Read the model definition and answer for the solid it produces. Units are mm, in the model's axes. A direction names the side the tool comes from. Round coordinates to 2 decimals unless told otherwise and drop trailing zeros. Order: outer loops, then holes, each group sorted by start corner. A loop starts at its lowest first (then second) coordinate and runs counter-clockwise, first axis right, second up. Notation, with made-up numbers: M 45,5 L 89,5 A13 ccw 89,9 Z; hole C 33.25,41 d8. An arc over 180 degrees is marked long. Answer as CSV lines item,"result".
```python
from build123d import *

# Parameters (mm, degrees)
SKETCH_1_W          = 36
SKETCH_1_H          = 15
EXTRUDE_1_DEPTH     = 4
SKETCH_2_W          = 36
SKETCH_2_H          = 3
EXTRUDE_2_DEPTH     = 10
SKETCH_3_R          = 1.7
CUT_EXTRUDE_1_DEPTH = 8
CHAMFER_1_SIZE      = 2
FILLET_1_R          = 0.5
FILLET_2_R          = 0.5


with BuildPart() as part:
    # Эскиз1 → Бобышка-Вытянуть1 (new body)
    with BuildSketch(Plane(origin=(0, 0, 0), x_dir=(1, 0, 0), z_dir=(0, 1, 0))):
        Rectangle(SKETCH_1_W, SKETCH_1_H)
    extrude(amount=EXTRUDE_1_DEPTH)

    # Эскиз2 → Бобышка-Вытянуть2 (add)
    with BuildSketch(Plane(origin=(0, 4, 0), x_dir=(1, 0, 0), z_dir=(0, 1, 0))):
        with Locations((0, 6)):
            Rectangle(SKETCH_2_W, SKETCH_2_H)
    extrude(amount=EXTRUDE_2_DEPTH)

    # Эскиз3 → Вырез-Вытянуть1 (cut)
    with BuildSketch(Plane.XZ):
        with Locations(Location((15, 0, 0), (0, 0, 270))):
            Circle(SKETCH_3_R)
        with Locations(Location((-15, 0, 0), (0, 0, 270))):
            Circle(SKETCH_3_R)
    extrude(amount=-CUT_EXTRUDE_1_DEPTH, mode=Mode.SUBTRACT)

    # Фаска1
    # the kernel refuses this chamfer: 2 mm, written as the material it takes off along each edge
    with BuildSketch(Plane(origin=(15, 0, 0), x_dir=(0, 0, -1), z_dir=(-1, 0, 0))) as chamfer_1_piece_1:
        Polygon((1.7 + CHAMFER_1_SIZE, 0), (1.7, -CHAMFER_1_SIZE), (1.7, 0), align=None)
    revolve(axis=Axis((15, 0, 0), (0, -1, 0)), mode=Mode.SUBTRACT)
    with BuildSketch(Plane(origin=(-15, 0, 0), x_dir=(0, 0, -1), z_dir=(-1, 0, 0))) as chamfer_1_piece_2:
        Polygon((1.7 + CHAMFER_1_SIZE, 0), (1.7, -CHAMFER_1_SIZE), (1.7, 0), align=None)
    revolve(axis=Axis((-15, 0, 0), (0, -1, 0)), mode=Mode.SUBTRACT)
    with BuildSketch(Plane(origin=(-23.143365976, 0, 7.5), x_dir=(0, 0.9996219169112968, 0.027495876610586494), z_dir=(1, 0, 0))) as chamfer_1_piece_3:
        Polygon((CHAMFER_1_SIZE * 0.999621916911, -CHAMFER_1_SIZE * 0.0274958766106), (-CHAMFER_1_SIZE * 0.0274958766106, -CHAMFER_1_SIZE * 0.999621916911), (0, 0), align=None)
    extrude(amount=46.286731952, mode=Mode.SUBTRACT)
    with BuildSketch(Plane(origin=(-18, 0, -12.643365976), x_dir=(-0.02749587661058563, 0.9996219169112968, 0), z_dir=(0, 0, 1)), Plane(origin=(18, 0, 12.643365976), x_dir=(0.02749587661058563, 0.9996219169112968, 0), z_dir=(0, 0, -1))) as chamfer_1_piece_4:
        Polygon((CHAMFER_1_SIZE * 0.999621916911, -CHAMFER_1_SIZE * 0.0274958766106), (-CHAMFER_1_SIZE * 0.0274958766106, -CHAMFER_1_SIZE * 0.999621916911), (0, 0), align=None)
    extrude(amount=25.286731952, mode=Mode.SUBTRACT)
    with BuildSketch(Plane(origin=(23.143365976, 0, -7.5), x_dir=(0, -0.027495876610586365, 0.9996219169112968), z_dir=(-1, 0, 0))) as chamfer_1_piece_5:
        Polygon((CHAMFER_1_SIZE * 0.999621916911, CHAMFER_1_SIZE * 0.0274958766106), (-CHAMFER_1_SIZE * 0.0274958766106, CHAMFER_1_SIZE * 0.999621916911), (0, 0), align=None)
    extrude(amount=46.286731952, mode=Mode.SUBTRACT)

    # Скругление1
    # the kernel refuses this fillet: 0.5 mm, written as the material it takes off along each edge
    with BuildSketch(Plane(origin=(-17.5, 13.5, -5), x_dir=(0, 0, 1), z_dir=(0, 1, 0))) as fillet_1_piece_1_section:
        Polygon((0, 0), (FILLET_1_R, 0), (FILLET_1_R, -FILLET_1_R), (0, -FILLET_1_R), align=None)
    fillet_1_piece_1 = extrude(amount=FILLET_1_R, mode=Mode.PRIVATE)
    fillet_1_piece_1 = fillet_1_piece_1 - Plane(origin=(-17.5, 13.5, -5), x_dir=(0.7071067811865475, 0, -0.7071067811865475), z_dir=(0, 1, 0)) * Sphere(FILLET_1_R, mode=Mode.PRIVATE)
    add(fillet_1_piece_1, mode=Mode.SUBTRACT)
    with BuildSketch(Plane(origin=(17.5, 13.5, -5), x_dir=(1, 0, 0), z_dir=(0, 1, 0))) as fillet_1_piece_2_section:
        Polygon((0, 0), (FILLET_1_R, 0), (FILLET_1_R, -FILLET_1_R), (0, -FILLET_1_R), align=None)
    fillet_1_piece_2 = extrude(amount=FILLET_1_R, mode=Mode.PRIVATE)
    fillet_1_piece_2 = fillet_1_piece_2 - Plane(origin=(17.5, 13.5, -5), x_dir=(-0.7071067811865475, 0, -0.7071067811865475), z_dir=(0, 1, 0)) * Sphere(FILLET_1_R, mode=Mode.PRIVATE)
    add(fillet_1_piece_2, mode=Mode.SUBTRACT)
    with BuildSketch(Plane(origin=(-17.5, 13.5, -7), x_dir=(0, 1, 0), z_dir=(0, 0, -1))) as fillet_1_piece_3_section:
        Polygon((0, 0), (FILLET_1_R, 0), (FILLET_1_R, -FILLET_1_R), (0, -FILLET_1_R), align=None)
    fillet_1_piece_3 = extrude(amount=FILLET_1_R, mode=Mode.PRIVATE)
    fillet_1_piece_3 = fillet_1_piece_3 - Plane(origin=(-17.5, 13.5, -7), x_dir=(0.7071067811865475, -0.7071067811865475, 0), z_dir=(0, 0, -1)) * Sphere(FILLET_1_R, mode=Mode.PRIVATE)
    add(fillet_1_piece_3, mode=Mode.SUBTRACT)
    with BuildSketch(Plane(origin=(17.5, 13.5, -7), x_dir=(0, 1, 0), z_dir=(0, 0, -1))) as fillet_1_piece_4_section:
        Polygon((0, 0), (FILLET_1_R, 0), (FILLET_1_R, FILLET_1_R), (0, FILLET_1_R), align=None)
    fillet_1_piece_4 = extrude(amount=FILLET_1_R, mode=Mode.PRIVATE)
    fillet_1_piece_4 = fillet_1_piece_4 - Plane(origin=(17.5, 13.5, -7), x_dir=(-0.7071067811865475, -0.7071067811865475, 0), z_dir=(0, 0, -1)) * Sphere(FILLET_1_R, mode=Mode.PRIVATE)
    add(fillet_1_piece_4, mode=Mode.SUBTRACT)
    with BuildSketch(Plane(origin=(-18, 4, -4.5), x_dir=(1, 0, 0), z_dir=(0, 0, 1))) as fillet_1_piece_5:
        with BuildLine():
            CenterArc((FILLET_1_R, -FILLET_1_R), FILLET_1_R, 90, 90)
            Line((0, -FILLET_1_R), (0, 0))
            Line((0, 0), (FILLET_1_R, 0))
        make_face()
    extrude(amount=13.25, mode=Mode.SUBTRACT)
    with BuildSketch(Plane(origin=(-18, 4, -4.5), x_dir=(0, 0, -1), z_dir=(0, 1, 0))) as fillet_1_piece_6:
        with BuildLine():
            CenterArc((FILLET_1_R, -FILLET_1_R), FILLET_1_R, 90, 90)
            Line((0, -FILLET_1_R), (0, 0))
            Line((0, 0), (FILLET_1_R, 0))
        make_face()
    extrude(amount=9.5, mode=Mode.SUBTRACT)
    with BuildSketch(Plane(origin=(18, 4, -4.5), x_dir=(0, 0, -1), z_dir=(0, 1, 0))) as fillet_1_piece_7:
        with BuildLine():
            CenterArc((FILLET_1_R, FILLET_1_R), FILLET_1_R, 180, 90)
            Line((0, FILLET_1_R), (0, 0))
            Line((0, 0), (FILLET_1_R, 0))
        make_face()
    extrude(amount=9.5, mode=Mode.SUBTRACT)
    with BuildSketch(Plane(origin=(-18, 14, -5), x_dir=(0, -1, 0), z_dir=(0, 0, -1)), Plane(origin=(18, 14, -7), x_dir=(0, -1, 0), z_dir=(0, 0, 1))) as fillet_1_piece_8:
        with BuildLine():
            CenterArc((FILLET_1_R, -FILLET_1_R), FILLET_1_R, 90, 90)
            Line((0, -FILLET_1_R), (0, 0))
            Line((0, 0), (FILLET_1_R, 0))
        make_face()
    extrude(amount=2, mode=Mode.SUBTRACT)
    with BuildSketch(Plane(origin=(17.5, 14, -4.5), x_dir=(0, 0, -1), z_dir=(-1, 0, 0))) as fillet_1_piece_9:
        with BuildLine():
            CenterArc((FILLET_1_R, FILLET_1_R), FILLET_1_R, 180, 90)
            Line((0, FILLET_1_R), (0, 0))
            Line((0, 0), (FILLET_1_R, 0))
        make_face()
    extrude(amount=35, mode=Mode.SUBTRACT)
    with BuildSketch(Plane(origin=(-17.5, 14, -7.5), x_dir=(0, -1, 0), z_dir=(1, 0, 0))) as fillet_1_piece_10:
        with BuildLine():
            CenterArc((FILLET_1_R, -FILLET_1_R), FILLET_1_R, 90, 90)
            Line((0, -FILLET_1_R), (0, 0))
            Line((0, 0), (FILLET_1_R, 0))
        make_face()
    extrude(amount=35, mode=Mode.SUBTRACT)
    with BuildSketch(Plane(origin=(-18, 2, -8.017766953), x_dir=(0, 1, 0), z_dir=(0, 0, 1)), Plane(origin=(18, 2, 8.017766953), x_dir=(0, 1, 0), z_dir=(0, 0, -1))) as fillet_1_piece_11:
        with BuildLine():
            CenterArc((FILLET_1_R * 0.414213562373, -FILLET_1_R), FILLET_1_R, 90, 45)
            Line((-FILLET_1_R * 0.292893218814, -FILLET_1_R * 0.292893218814), (0, 0))
            Line((0, 0), (FILLET_1_R * 0.414213562373, 0))
        make_face()
    extrude(amount=16.035533906, mode=Mode.SUBTRACT)
    with BuildSketch(Plane(origin=(18, 4, 8.75), x_dir=(0, -1, 0), z_dir=(0, 0, -1))) as fillet_1_piece_12:
        with BuildLine():
            CenterArc((FILLET_1_R, FILLET_1_R), FILLET_1_R, 180, 90)
            Line((0, FILLET_1_R), (0, 0))
            Line((0, 0), (FILLET_1_R, 0))
        make_face()
    extrude(amount=13.25, mode=Mode.SUBTRACT)
    with BuildSketch(Plane(origin=(18, 0.75, 7.5), x_dir=(-1, 0, 0), z_dir=(0, 1, 0))) as fillet_1_piece_13:
        with BuildLine():
            CenterArc((FILLET_1_R, -FILLET_1_R), FILLET_1_R, 90, 90)
            Line((0, -FILLET_1_R), (0, 0))
            Line((0, 0), (FILLET_1_R, 0))
        make_face()
    extrude(amount=4.5, mode=Mode.SUBTRACT)
    with BuildSketch(Plane(origin=(-18, 0.75, 7.5), x_dir=(1, 0, 0), z_dir=(0, 1, 0))) as fillet_1_piece_14:
        with BuildLine():
            CenterArc((FILLET_1_R, FILLET_1_R), FILLET_1_R, 180, 90)
            Line((0, FILLET_1_R), (0, 0))
            Line((0, 0), (FILLET_1_R, 0))
        make_face()
    extrude(amount=4.5, mode=Mode.SUBTRACT)
    with BuildSketch(Plane(origin=(-18, 13.5, -7.5), x_dir=(0, 0, 1), z_dir=(0, -1, 0)), Plane(origin=(18, 0.75, -7.5), x_dir=(0, 0, 1), z_dir=(0, 1, 0))) as fillet_1_piece_15:
        with BuildLine():
            CenterArc((FILLET_1_R, -FILLET_1_R), FILLET_1_R, 90, 90)
            Line((0, -FILLET_1_R), (0, 0))
            Line((0, 0), (FILLET_1_R, 0))
        make_face()
    extrude(amount=12.75, mode=Mode.SUBTRACT)
    with BuildSketch(Plane(origin=(-18, 4, -5.75), x_dir=(1, 0, 0), z_dir=(0, 0, 1))) as fillet_1_piece_16a_section:
        with BuildLine():
            CenterArc((FILLET_1_R, -FILLET_1_R), FILLET_1_R, 90, 90)
            Line((0, -FILLET_1_R), (0, 0))
            Line((0, 0), (FILLET_1_R, 0))
        make_face()
    fillet_1_piece_16a = extrude(amount=14.5, mode=Mode.PRIVATE)
    fillet_1_piece_16a = split(fillet_1_piece_16a, bisect_by=Plane(origin=(-17.886802443, 3.886802443, -4.5), z_dir=(0, 0, -1)), keep=Keep.TOP, mode=Mode.PRIVATE)
    with BuildSketch(Plane(origin=(-18, 2.75, -4.5), x_dir=(0, 0, -1), z_dir=(0, 1, 0))) as fillet_1_piece_16b_section:
        with BuildLine():
            CenterArc((FILLET_1_R, -FILLET_1_R), FILLET_1_R, 90, 90)
            Line((0, -FILLET_1_R), (0, 0))
            Line((0, 0), (FILLET_1_R, 0))
        make_face()
    fillet_1_piece_16b = extrude(amount=10.75, mode=Mode.PRIVATE)
    fillet_1_piece_16b = split(fillet_1_piece_16b, bisect_by=Plane(origin=(-17.886802443, 4, -4.613197557), z_dir=(0, -1, 0)), keep=Keep.TOP, mode=Mode.PRIVATE)
    fillet_1_piece_16 = fillet_1_piece_16a & fillet_1_piece_16b
    add(fillet_1_piece_16, mode=Mode.SUBTRACT)
    with BuildSketch(Plane(origin=(18, 2.75, -4.5), x_dir=(0, 0, -1), z_dir=(0, 1, 0))) as fillet_1_piece_17a_section:
        with BuildLine():
            CenterArc((FILLET_1_R, FILLET_1_R), FILLET_1_R, 180, 90)
            Line((0, FILLET_1_R), (0, 0))
            Line((0, 0), (FILLET_1_R, 0))
        make_face()
    fillet_1_piece_17a = extrude(amount=10.75, mode=Mode.PRIVATE)
    fillet_1_piece_17a = split(fillet_1_piece_17a, bisect_by=Plane(origin=(17.886802443, 4, -4.613197557), z_dir=(0, -1, 0)), keep=Keep.TOP, mode=Mode.PRIVATE)
    with BuildSketch(Plane(origin=(18, 4, 8.75), x_dir=(0, -1, 0), z_dir=(0, 0, -1))) as fillet_1_piece_17b_section:
        with BuildLine():
            CenterArc((FILLET_1_R, FILLET_1_R), FILLET_1_R, 180, 90)
            Line((0, FILLET_1_R), (0, 0))
            Line((0, 0), (FILLET_1_R, 0))
        make_face()
    fillet_1_piece_17b = extrude(amount=14.5, mode=Mode.PRIVATE)
    fillet_1_piece_17b = split(fillet_1_piece_17b, bisect_by=Plane(origin=(17.886802443, 3.886802443, -4.5), z_dir=(0, 0, -1)), keep=Keep.TOP, mode=Mode.PRIVATE)
    fillet_1_piece_17 = fillet_1_piece_17a & fillet_1_piece_17b
    add(fillet_1_piece_17, mode=Mode.SUBTRACT)

    # Скругление2
    # the kernel refuses this fillet: 0.5 mm, written as the material it takes off along each edge
    with BuildSketch(Plane(origin=(17.5, 3.5, 7), x_dir=(0, 1, 0), z_dir=(0, 0, 1))) as fillet_2_piece_1_section:
        Polygon((0, 0), (FILLET_2_R, 0), (FILLET_2_R, -FILLET_2_R), (0, -FILLET_2_R), align=None)
    fillet_2_piece_1 = extrude(amount=FILLET_2_R, mode=Mode.PRIVATE)
    fillet_2_piece_1 = fillet_2_piece_1 - Plane(origin=(17.5, 3.5, 7), x_dir=(-0.7071067811865475, -0.7071067811865475, 0), z_dir=(0, 0, 1)) * Sphere(FILLET_2_R, mode=Mode.PRIVATE)
    add(fillet_2_piece_1, mode=Mode.SUBTRACT)
    with BuildSketch(Plane(origin=(-17.5, 3.5, 7), x_dir=(0, 1, 0), z_dir=(0, 0, 1))) as fillet_2_piece_2_section:
        Polygon((0, 0), (FILLET_2_R, 0), (FILLET_2_R, FILLET_2_R), (0, FILLET_2_R), align=None)
    fillet_2_piece_2 = extrude(amount=FILLET_2_R, mode=Mode.PRIVATE)
    fillet_2_piece_2 = fillet_2_piece_2 - Plane(origin=(-17.5, 3.5, 7), x_dir=(0.7071067811865475, -0.7071067811865475, 0), z_dir=(0, 0, 1)) * Sphere(FILLET_2_R, mode=Mode.PRIVATE)
    add(fillet_2_piece_2, mode=Mode.SUBTRACT)
    with BuildSketch(Plane(origin=(-17.5, 4, 7.5), x_dir=(0, -1, 0), z_dir=(1, 0, 0))) as fillet_2_piece_3:
        with BuildLine():
            CenterArc((FILLET_2_R, FILLET_2_R), FILLET_2_R, 180, 90)
            Line((0, FILLET_2_R), (0, 0))
            Line((0, 0), (FILLET_2_R, 0))
        make_face()
    extrude(amount=35, mode=Mode.SUBTRACT)


solid = part.part
```
Item 1: A cutting plane is placed at C-C, the plane z = 4.75. Determine the outline of the cut face in (x, y), and give its area (3 significant figures).
Ans:
outline,"M -18,2.21 A0.5 ccw -17.85,1.85 L -16,0 L 16,0 L 17.85,1.85 A0.5 ccw 18,2.21 L 18,3.5 A0.5 ccw 17.5,4 L -17.5,4 A0.5 ccw -18,3.5 Z"
area,"140 mm2"
Item 2: Find the intervals of material crossed by probe 1 along X at (y, z) = (2.75, 0); probe 2 along Y at (x, z) = (0, -1.5); probe 3 along Z at (x, y) = (10, 12), in increasing order. Write a range as [from, to].
Ans:
probe 1,"[-18, -16.7], [-13.3, 13.3], [16.7, 18]"
probe 2,"[0, 4]"
probe 3,"[-7.5, -4.5]"
Item 3: Flat-ended cylindrical pins translate along their axes: pin 1 (3.5 mm diameter, centred on x = -4, z = -0.5, fed in from +Y); pin 2 (2 mm diameter, centred on x = 10, y = 9, fed in from +Z). Find the tip coordinate at first contact, or state that the pin passes through.
Ans:
pin 1,"y = 4"
pin 2,"z = -4.5"
Item 4: A cutting plane is placed at A-A, the plane z = 0. Determine the outline of the cut face in (x, y).
Ans:
outline,"M -18,2.21 A0.5 ccw -17.85,1.85 L -17.35,1.35 L -16.7,2 L -16.7,4 L -17.5,4 A0.5 ccw -18,3.5 Z; M -13.3,2 L -11.3,0 L 11.3,0 L 13.3,2 L 13.3,4 L -13.3,4 Z; M 16.7,2 L 17.35,1.35 L 17.85,1.85 A0.5 ccw 18,2.21 L 18,3.5 A0.5 ccw 17.5,4 L 16.7,4 Z"
Item 5: A cutting plane is placed at B-B, the plane x = 15. Determine the outline of the cut face in (y, z), and give its area (3 significant figures).
Ans:
outline,"M 0,-5.5 L 2,-7.5 L 13.5,-7.5 A0.5 ccw 14,-7 L 14,-5 A0.5 ccw 13.5,-4.5 L 4,-4.5 L 4,-1.7 L 2,-1.7 L 0,-3.7 Z; M 0,3.7 L 2,1.7 L 4,1.7 L 4,7 A0.5 ccw 3.5,7.5 L 2,7.5 L 0,5.5 Z"
area,"68.2 mm2"
Item 6: A cutting plane is placed at D-D, the plane y = 6.5. Determine the outline of the cut face in (x, z).
Ans:
outline,"M -18,-7 A0.5 ccw -17.5,-7.5 L 17.5,-7.5 A0.5 ccw 18,-7 L 18,-5 A0.5 ccw 17.5,-4.5 L -17.5,-4.5 A0.5 ccw -18,-5 Z"
Item 7: Determine the mould class of faces 3 (the face through (13.03, 1.68, 0.44)), 4 (the face through (18, 5.7, -5.2)), 5 (the face through (0, 14, -6)), 6 (the face through (-18, 5.7, -5.2)) for opening direction X: +X half, -X half, draft (parallel to the pull), parting line (faces both ways), or undercut.
Ans:
face 3,"undercut"
face 4,"+X half"
face 5,"draft"
face 6,"-X half"
Item 8: A tool of negligible diameter and unlimited length cuts with its end or side. For faces 1 (the face through (0, 4, 1)), 2 (the face through (0, 8, -7.5)), from which of +Z, -Z, +X, -X, +Y, -Y can it reach the whole face along a straight path? Write none if from no direction.
Ans:
face 1,"+Z, +X, -X, +Y"
face 2,"-Z, +X, -X, +Y, -Y"
